from build123d import *

# Parameters (mm, degrees)
SKETCH1_R           = 2.5
BOSS_EXTRUDE1_DEPTH = 5


with BuildPart() as part:
    # Sketch1 → Boss-Extrude1 (new body)
    with BuildSketch(Plane(origin=(0, 0, 0), x_dir=(0, 0, -1), z_dir=(1, 0, 0))):
        with BuildLine():
            Line((32.973972115, 3.535533906), (59.8440298, -23.334523779))
            ThreePointArc((59.8440298, -23.334523779), (59.8440298, -30.405591591), (52.772961988, -30.405591591))
            Line((52.772961988, -30.405591591), (25.902904303, -3.535533906))
            ThreePointArc((25.902904303, -3.535533906), (25.902904303, 3.535533906), (32.973972115, 3.535533906))
        make_face()
        with Locations((29.438438209, 0)):
            Circle(SKETCH1_R, mode=Mode.SUBTRACT)
        with Locations((56.323505195, -26.885066985)):
            Circle(SKETCH1_R, mode=Mode.SUBTRACT)
    extrude(amount=BOSS_EXTRUDE1_DEPTH)


solid = part.part
Verification items for the finished model (mm, model axes). Give positions to 0.01 mm unless a question says otherwise; leave off trailing zeros. Write each loop counter-clockwise with the first axis right and the second up, starting at its lowest first coordinate (ties: lowest second). Pieces come first, ordered by that corner, then holes. Notation, with made-up numbers: M 28.5,-16 L 83.5,-16 A20 ccw 83.5,18 Z; hole C -25.5,88 d11. An arc over 180 degrees is marked long. Put each result on its own line as item: value. Start each with the question number.
1. Go/stop test with flat-tipped pins: pin 1 Ø1.5 at (x, z) = (4, -51.5) entering from +Y; pin 2 Ø3 at (x, z) = (1, -32.5) entering from +Y; pin 3 Ø5 at (y, z) = (-17, -34.5) entering from -X; pin 4 Ø1 at (x, y) = (2, -7.5) entering from +Z. Record where each tip stops, or that it passes through.
2. Section check C-C (x = 3.65). Record the cut outline in (y, z), and give its area (3 significant figures).
3. Section check D-D (z = -51). Record the cut outline in (x, y), and give its area (3 significant figures).
4. Section check B-B (y = 0). Record the cut outline in (x, z).
5. Scan lines: line 1 along Y through (x, z) = (0.35, -27.5); line 2 along Y through (x, z) = (1.6, -28); line 3 along Z through (x, y) = (1.85, 1.5). Record each from-to range of solid material in increasing order. Write a range as [from, to].
6. Section check A-A (z = -28). Record the cut outline in (x, y).
7. Draft check along Z on faces 1 (the face through (2.465, 0.751, -31.823)), 2 (the face through (2.465, -26.775, -53.826)), 3 (the face through (2.46, -9.71, -46.22)), 4 (the face through (2.46, -17.16, -39.53)). Enter one of: +Z half, -Z half, draft (parallel to the pull), parting line (faces both ways), or undercut.
Answer list:
1. pin 1: y = -14.24
1. pin 2: y = 4.75
1. pin 3: through
1. pin 4: z = -29.37
2. outline: M -30.41,-52.77 A5 ccw -23.33,-59.84 L 3.54,-32.97 A5 ccw -3.54,-25.9 Z; hole C -26.89,-56.32 d5; hole C 0,-29.44 d5
2. area: 419 mm2
3. outline: M 0,-28.63 L 5,-28.63 L 5,-14.49 L 0,-14.49 Z
3. area: 70.7 mm2
4. outline: M 0,-36.51 L 5,-36.51 L 5,-31.94 L 0,-31.94 Z; M 0,-26.94 L 5,-26.94 L 5,-24.44 L 0,-24.44 Z
5. line 1: [-5.13, -1.58], [1.58, 4.61]
5. line 2: [-5.63, -2.04], [2.04, 4.79]
5. line 3: [-35.01, -31.44], [-27.44, -24.67]
6. outline: M 0,-5.63 L 5,-5.63 L 5,-2.04 L 0,-2.04 Z; M 0,2.04 L 5,2.04 L 5,4.79 L 0,4.79 Z
7. face 1: undercut
7. face 2: undercut
7. face 3: -Z half
7. face 4: +Z half
